The listing builds one solid part. Answer for the finished solid, in the listing's coordinates (mm). Face numbers are marked on the shaded views. A direction names the side the tool comes from. Round coordinates to 2 decimals unless told otherwise and drop trailing zeros. Order: outer loops, then holes, each group sorted by start corner. A loop starts at its lowest first (then second) coordinate and runs counter-clockwise, first axis right, second up. Notation, with made-up numbers: (-25.5, 68) -> (21.5, 68) arc R22 ccw to (21.5, 106) -> close; hole circle Ø7 at (10, -39.75). An arc over 180 degrees is marked (long way). Answer in a Markdown table with one row per item. Add a question column.
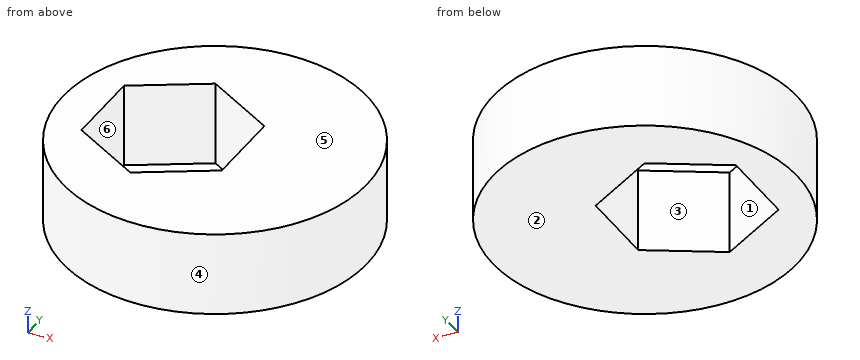
```python
from build123d import *

# Parameters (mm, degrees)
SKETCH1_R           = 10.85
BOSS_EXTRUDE1_DEPTH = 6


with BuildPart() as part:
    # Sketch1 → Boss-Extrude1 (new body)
    with BuildSketch(Plane.XY):
        with Locations((3, 0)):
            Circle(SKETCH1_R)
        Polygon((0, 5.773502692), (-5, 2.886751346), (-5, -2.886751346), (0, -5.773502692), (5, -2.886751346), (5, 2.886751346), align=None, mode=Mode.SUBTRACT)
    extrude(amount=-BOSS_EXTRUDE1_DEPTH)


solid = part.part
```
1. The mould has two halves that part along X. Classify the marked faces 3, 4, 5 and 6: released by +X, released by -X, zero draft, split by the parting line, or undercut.
2. The part is cut by section A-A (y = 0). Give the vertices of the cut face in (x, z).
3. The part is cut by section B-B (z = -4.9). Give the vertices of the cut face in (x, y).
4. Straight lines are drawn through the part: line 1 along X through (y, z) = (5.5, -2.6); line 2 along X through (y, z) = (4.25, -4.8); line 3 along Y through (x, z) = (3, -2.55). For each, find the intervals that lie inside material, in ascending order.
5. The part is cut by section C-C (x = 0.5). Give the vertices of the cut face in (y, z).
6. Each of these flat-tipped pins is pushed along its axis until it touches: pin 1 (2 mm diameter, centred on x = 8, z = -5.5, fed in from -Y); pin 2 (1 mm diameter, centred on x = 6, y = -2, fed in from +Z); pin 3 (3 mm diameter, centred on y = 7.5, z = -2, fed in from -X). Where does it stop, or does it pass through?
7. The part is cut by section D-D (x = 9.5). Give the vertices of the cut face in (y, z).
8. For the marked faces 1 and 2, determine the directions among +Z, -Z, +X, -X, +Y, -Y from which every point of the face is accessible in a straight line to the end or side of a thin tool.
Report:
| question | item | result |
|---|---|---|
| 1 | face 3 | undercut |
| 1 | face 4 | split by the parting line |
| 1 | face 5 | zero draft |
| 1 | face 6 | undercut |
| 2 | outline | (-7.85, -6) -> (-5, -6) -> (-5, 0) -> (-7.85, 0) -> close; (5, -6) -> (13.85, -6) -> (13.85, 0) -> (5, 0) -> close |
| 3 | outline | circle Ø21.7 at (3, 0); hole (-5, -2.89) -> (0, -5.77) -> (5, -2.89) -> (5, 2.89) -> (0, 5.77) -> (-5, 2.89) -> close |
| 4 | line 1 | x = -6.35 to -0.47, 0.47 to 12.35 |
| 4 | line 2 | x = -6.98 to -2.64, 2.64 to 12.98 |
| 4 | line 3 | y = -10.85 to -4.04, 4.04 to 10.85 |
| 5 | outline | (-10.56, -6) -> (-5.48, -6) -> (-5.48, 0) -> (-10.56, 0) -> close; (5.48, -6) -> (10.56, -6) -> (10.56, 0) -> (5.48, 0) -> close |
| 6 | pin 1 | stops at y = -10.09 |
| 6 | pin 2 | stops at z = 0 |
| 6 | pin 3 | stops at x = -6.04 |
| 7 | outline | (-8.69, -6) -> (8.69, -6) -> (8.69, 0) -> (-8.69, 0) -> close |
| 8 | face 1 | +Z, -Z |
| 8 | face 2 | -Z, +X, -X, +Y, -Y |
